Read the model definition and answer for the solid it produces. Units are mm, in the model's axes. A direction names the side the tool comes from. Coordinates: 2 decimals unless noted, no trailing zeros. Write each loop counter-clockwise with the first axis right and the second up, starting at its lowest first coordinate (ties: lowest second). Pieces come first, ordered by that corner, then holes. Notation, with made-up numbers: (25, -14) -> (62, -14) arc R34 cw to (62, 17) -> close; hole circle Ø3 at (86.5, -3). An arc over 180 degrees is marked (long way). One line per item, written item: value. Start each with the question number.
1. For a pull along Z with two mould halves and no side action, classify faces 3 (the cylindrical face through (0.21, 409.54, -227)), 4 (the flat face through (0, -700, 0)), 5 (the flat face through (0, 400, 250)) as pulls with the +Z half, pulls with the -Z half, needs draft (parallel to the pull), parting line crosses it, or undercut.
2. Find section A-A, the plane z = -230. Write down the section's boundary in (x, y), and give its area (3 significant figures).
3. Find section C-C, the plane z = -137. Write down the section's boundary in (x, y), and give its area (3 significant figures).
4. Find section B-B, the plane y = 74.5. Write down the section's boundary in (x, z).
5. Given P1, Ø4, axis at x = 2, y = -491, coming from the -Z side; P2, Ø12, axis at x = 2, z = 166, coming from the +Y side; P3, Ø1, axis at x = -0.5, z = 59, coming from the -Y side; P4, Ø1.5, axis at x = 8, y = -572, coming from the +Z side, each flat-ended and moving along its own axis, determine where each tip first touches the part or whether it passes through.
6. Consider line 1 along Z through (x, y) = (8.5, 400); line 2 along Z through (x, y) = (-1.5, 137.5); line 3 along Y through (x, z) = (11, 156). Determine where each line is inside the solid, lowest interval first.
7. For faces 1 (the cylindrical face through (0.21, 409.54, 233)), 2 (the cylindrical face through (-3.252, 414.643, -3.5)), determine the directions among +Z, -Z, +X, -X, +Y, -Y from which every point of the face is accessible in a straight line to the end or side of a thin tool.
Autodesk Inventor part; units mm, degrees
ref_plane "Płaszczyzna konstrukcyjna1" through (15, 0, 0) normal (1, 0, 0) x (0, 1, 0)
ref_plane "XZ Plane" through (0, 0, 0) normal (0, 1, 0) x (-1, 0, 0)
ref_plane "XY Plane" through (0, 0, 0) normal (0, 0, 1) x (1, 0, 0)
sketch "Szkic1" plane through (0, 0, 0) normal (0, 1, 0) x (-1, 0, 0)
  circle A0 centre (0, 0) radius 15
  dimension "d0" = 30
extrude "Wyciągnięcie proste1" add sketch "Szkic1" along normal blind 400
sketch "Szkic2" plane through (0, 0, 0) normal (0, 0, 1) x (1, 0, 0)
  point P0 (0, 0)
sketch "Szkic3" plane through (0, 0, 0) normal (0, 0, 1) x (1, 0, 0)
  circle A0 centre (0, 400) radius 15
  point P0 (0, 0)
  dimension "d3" = 30
extrude "Wyciągnięcie proste2" add sketch "Szkic3" along normal mid plane 500
fillet "Zaokrąglenie1" radius 4 4 edges at (-10.6066, 389.3934, -10.6066) (10.6066, 389.3934, -10.6066) (10.6066, 389.3934, 10.6066) (-10.6066, 389.3934, 10.6066)
ref_plane "Płaszczyzna konstrukcyjna1" through (15, 0, 0) normal (1, 0, 0) x (0, 1, 0)
sketch "Szkic4" plane through (15, 0, 0) normal (1, 0, 0) x (0, 1, 0)
  line L0 (400, 0) -> (400, 0)
  line L1 (400, 0) -> (400, 0)
  line L2 (415, 250) -> (385, 250)
  line L3 (385, -250) -> (415, -250)
  line L4 (400, 0) -> (400, 0)
  line L5 (400, 0) -> (400, 0)
  line L6 (0, 15) -> (0, -15)
  line L7 (0, 15) -> (381, 15)
  line L8 (0, -15) -> (381, -15)
  line L9 (385, -250) -> (385, 250)
  line L10 (415, -250) -> (415, 250)
  circle A0 centre (400, 230) radius 10
  point P0 (0, 0)
  dimension "d8" = 20
  dimension "d9" = 20
extrude "Wyciągnięcie proste3" cut sketch "Szkic4" against normal through all contours A0
mirror "Odbicie lustrzane1" about plane through (0, 0, 0) normal (0, 0, 1) of "Wyciągnięcie proste3"
sketch "Szkic5" plane through (0, 0, 0) normal (0, -1, 0) x (1, 0, 0)
  circle A0 centre (0, 0) radius 15
extrude "Wyciągnięcie proste4" add sketch "Szkic5" along normal blind 700
sketch "Szkic6" plane through (15, 0, 0) normal (1, 0, 0) x (0, 1, 0)
  point P0 (0, 0)
properties part number "1" material "Złote"
Answer block:
1. face 3: undercut
1. face 4: needs draft
1. face 5: pulls with the +Z half
2. outline: (-11.18, 390) arc R15 ccw to (11.18, 390) -> close; (-11.18, 410) -> (11.18, 410) arc R15 ccw to start
2. area: 155 mm2
3. outline: circle Ø30 at (0, 400)
3. area: 707 mm2
4. outline: circle Ø30 at (0, 0)
5. P1: stops at z = -15
5. P2: stops at y = 415
5. P3: stops at y = 385
5. P4: stops at z = 13.13
6. line 1: z = -250 to -240, -220 to 220, 240 to 250
6. line 2: z = -14.92 to 14.92
6. line 3: y = 389.8 to 410.2
7. face 1: +X, -X
7. face 2: none
